Autodesk Inventor part; units mm, degrees
ref_plane "YZ Plane" through (0, 0, 0) normal (1, 0, 0) x (0, 1, 0)
ref_plane "XZ Plane" through (0, 0, 0) normal (0, 1, 0) x (-1, 0, 0)
ref_plane "XY Plane" through (0, 0, 0) normal (0, 0, 1) x (1, 0, 0)
sketch "Sketch1" plane through (0, 0, 0) normal (1, 0, 0) x (0, 1, 0)
  line L0 (-13.4609, 51.6064) -> (11.5391, 51.6064)
  line L1 (11.5391, -50.3936) -> (-13.4609, -50.3936)
  line L2 (-13.4609, -50.3936) -> (-13.4609, 51.6064)
  line L3 (-13.4609, 51.6064) -> (11.5391, -50.3936) construction
  line L4 (11.5391, 51.6064) -> (-13.4609, -50.3936) construction
  line L5 (1.5391, 22.2064) -> (1.5391, -20.9936)
  line L6 (6.5391, 37.8564) -> (11.5391, 34.9696)
  line L7 (6.5391, -36.6436) -> (11.5391, -33.7569)
  line L8 (6.5391, -36.6436) -> (13.9505, -36.6436) construction
  line L9 (1.5391, 22.2064) -> (6.5391, 19.3196)
  line L10 (1.5391, -20.9936) -> (6.5391, -18.1069)
  line L11 (6.5391, 37.8564) -> (6.5391, 19.3196)
  line L12 (6.5391, -18.1069) -> (6.5391, -36.6436)
  line L13 (11.5391, 51.6064) -> (11.5391, 34.9696)
  line L14 (11.5391, -33.7569) -> (11.5391, -50.3936)
  point P0 (-0.9609, 0.6064)
  dimension "d2" = 25
  dimension "d3" = 102
  dimension "d4" = 43.2
  dimension "d5" = 21.6
  dimension "d6" = 74.5
  dimension "d7" = 37.25
  dimension "d10" = 30
extrude "Extrusion1" add sketch "Sketch1" along normal blind 203
sketch "Sketch2" plane through (0, 1.5391, 22.2064) normal (0, 1, 0) x (1, 0, 0)
  point P0 (0, 22.2064)
  point P1 (63.4, 22.2064)
  point P2 (139.6, 22.2064)
  dimension "d14" = 76.2
  dimension "d15" = 63.4
hole "Hole1" at (63.4, 1.5391, 0) at (139.6, 1.5391, 0) direction (0, -1, 0) diameter 8.4 end through all counterbore diameter 15 counterbore depth 9
sketch "Sketch3" plane through (0, 1.5391, 22.2064) normal (0, 1, 0) x (1, 0, 0)
  point P0 (0, 22.2064)
  point P1 (84, 22.2064)
  point P2 (119, 22.2064)
  dimension "d23" = 35
  dimension "d24" = 84
hole "Hole2" at (84, 1.5391, 0) at (119, 1.5391, 0) direction (0, -1, 0) diameter 8.4 end through all counterbore diameter 15 counterbore depth 9
sketch "Sketch4" plane through (0, -13.4609, 51.6064) normal (0, 0, 1) x (1, 0, 0)
  line L0 (0, 0) -> (203, 0)
  line L1 (0, 0) -> (0, 25)
  line L2 (203, 25) -> (203, 0)
  point P0 (0, 13.4609)
  point P1 (50, 12.5)
  point P2 (153, 12.5)
  dimension "d32" = 12.5
  dimension "d33" = 12.5
  dimension "d34" = 50
  dimension "d35" = 50
hole "Hole3" at (50, -0.9609, 51.6064) at (153, -0.9609, 51.6064) direction (0, 0, -1) diameter 10 depth 10 tip angle 118
properties part number "czescuchwytu" material "Iron, Cast"
Check sheet for the modelled part. Datum: model origin and axes. Units: mm. A direction names the side the tool comes from. Give positions to 0.01 mm unless a question says otherwise; leave off trailing zeros. Loops run counter-clockwise (first coordinate to the right, second up) from the corner with the lowest first, then second, coordinate; pieces in that order, holes last. Notation, with made-up numbers: M 17.25,74.5 L 72.25,74.5 A22 cw 72.25,97.5 Z; hole C 51.5,48.25 d11. An arc over 180 degrees is marked long. Return JSON: item names as keys, results as strings. Group by question number.
1. Tool access check on faces 1 (the flat face through (143, -7.461, 3)), 2 (the flat face through (100, 1.539, 1)), 3 (the flat face through (100, -1, 51.606)). Record the directions out of +Z, -Z, +X, -X, +Y, -Y that give a thin tool (end or side, any length) a straight path to the whole face; none if there is none.
2. Cross-section at B-B on x = 182. Record the boundary of the cut face in (y, z), plus the area to 3 significant figures.
3. Cross-section at C-C on z = 0. State how many separate pieces and enclosed holes the cut face has, plus the area to 3 significant figures.
4. Mould release check, pull along Z, two halves, no side actions. Record for faces 4 (the flat face through (100, 11.539, 43)), 5 (the flat face through (100, -1, -50.394)), 6 (the conical face through (152.152, -0.773, 39.124)), 7 (the cylindrical face through (126.32, -3.02, -1.63)): released by +Z, released by -Z, zero draft, split by the parting line, or undercut.
5. Cross-section at A-A on x = 119. Record the boundary of the cut face in (y, z).
6. Cross-section at D-D on z = -25. Record the boundary of the cut face in (x, y).
7. Thickness scan on L1, parallel to X at y = -1.25, z = 0; L2, parallel to X at y = -9, z = 0; L3, parallel to Z at x = 63.4, y = -0.5. Record the ranges inside material, lowest first.
8. Go/stop test with flat-tipped pins: pin 1 (16.5 mm diameter, centred on x = 63, z = -3.5, fed in from +Y); pin 2 (4.5 mm diameter, centred on x = 85.5, z = 3.5, fed in from +Y); pin 3 (5.5 mm diameter, centred on x = 111, z = 25, fed in from +Y); pin 4 (5 mm diameter, centred on x = 139.6, z = 0, fed in from -Y). Record where each tip stops, or that it passes through.
Return value:
{
 "1": {"face 1": "+Y", "face 2": "+X, -X", "face 3": "+Z, +X, -X, +Y, -Y"},
 "2": {"outline": "M -13.46,-50.39 L 11.54,-50.39 L 11.54,-33.76 L 6.54,-36.64 L 6.54,-18.11 L 1.54,-20.99 L 1.54,22.21 L 6.54,19.32 L 6.54,37.86 L 11.54,34.97 L 11.54,51.61 L -13.46,51.61 Z", "area": "1,990 mm^2"},
 "3": {"separate pieces": "5", "enclosed holes": "0", "area": "2,300 mm^2"},
 "4": {"face 4": "zero draft", "face 5": "released by -Z", "face 6": "released by +Z", "face 7": "undercut"},
 "5": {"outline": "M -13.46,-50.39 L 11.54,-50.39 L 11.54,-33.76 L 6.54,-36.64 L 6.54,-18.11 L 1.54,-20.99 L 1.54,-7.5 L -7.46,-7.5 L -7.46,-4.2 L -13.46,-4.2 Z; M -13.46,4.2 L -7.46,4.2 L -7.46,7.5 L 1.54,7.5 L 1.54,22.21 L 6.54,19.32 L 6.54,37.86 L 11.54,34.97 L 11.54,51.61 L -13.46,51.61 Z"},
 "6": {"outline": "M 0,-13.46 L 203,-13.46 L 203,6.54 L 0,6.54 Z"},
 "7": {"L1": "0 to 55.9, 70.9 to 76.5, 91.5 to 111.5, 126.5 to 132.1, 147.1 to 203", "L2": "0 to 59.2, 67.6 to 79.8, 88.2 to 114.8, 123.2 to 135.4, 143.8 to 203", "L3": "-50.39 to -7.5, 7.5 to 51.61"},
 "8": {"pin 1": "y = 1.54", "pin 2": "y = -7.46", "pin 3": "y = 6.54", "pin 4": "through"}
}
